Source: CAD feature listing. Evaluate the final solid. Frame: model axes, mm. Face numbers are marked on the shaded views. Coordinates: 2 decimals unless noted, no trailing zeros. Write each loop counter-clockwise with the first axis right and the second up, starting at its lowest first coordinate (ties: lowest second). Pieces come first, ordered by that corner, then holes. Notation, with made-up numbers: M 77,75.25 L 115,75.25 A26 cw 115,106.25 Z; hole C -4,-28 d7. An arc over 180 degrees is marked long. One line per item, written item: value. Start each with the question number.
Item 1: Cut plane B-B, the plane z = 1. Output: boundary loops of the cut face in (x, y), then the cut area to 3 significant figures.
Item 2: Cut plane A-A, the plane z = -19. Output: boundary loops of the cut face in (x, y).
Item 3: Pin query (flat end, axial travel): P1, Ø12, axis at x = -16, z = -2, coming from the -Y side; P2, Ø10, axis at y = -15, z = -2, coming from the -X side; P3, Ø5, axis at x = 0, y = 0, coming from the -Z side. Return the tip coordinate at first contact, or that it passes through.
Item 4: Ray query, L1, parallel to Y at x = 0, z = 22; L2, parallel to X at y = 0, z = 21.25; L3, parallel to X at y = 0, z = 18.25. Return the intervals inside material, ascending. Write a range as from..to.
Item 5: Mould query, pull axis X, two halves, no side actions, for the marked faces 1, 2, 3 and 4. Classes: released by +X, released by -X, zero draft, split by the parting line, or undercut.
Item 6: Cut plane C-C, the plane z = 10.5. Output: boundary loops of the cut face in (x, y), then the cut area to 3 significant figures.
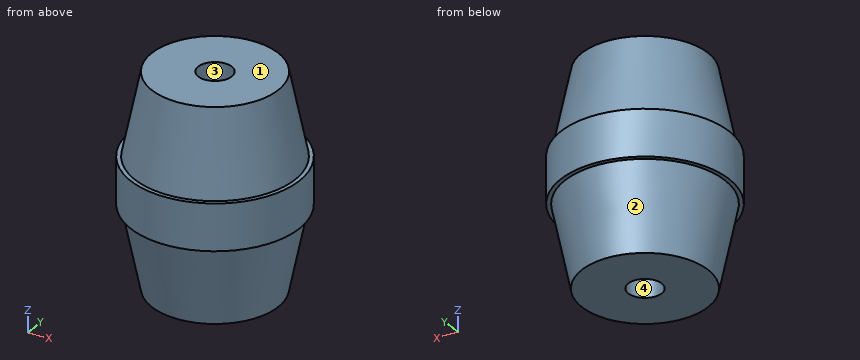
```python
from build123d import *

# Parameters (mm, degrees)
F4_D           = 8
F4_DEPTH       = 10
F4_TIP         = 2.4034424761
F4_ON_F2_D     = 8
F4_ON_F2_DEPTH = 10
F4_ON_F2_TIP   = 2.4034424761


with BuildPart() as f1:
    # F0 (on Front) → F1 (revolve)
    with BuildSketch(Plane.XZ):
        Polygon((0, -25), (0, 25), (-15, 25), (-19, 5.5), (-20, 5.5), (-20, 0), (-20, -5.5), (-20, -5.5145598017), (-19, -5.5145598017), (-15, -25), align=None)
    revolve(axis=Axis((0, 0, 0), (0, 0, -1)))

    # F4
    with Locations(Plane(origin=(0, 0, -25), x_dir=(1, 0, 0), z_dir=(0, 0, -1))):
        with Locations((0, 0)):
            Hole(F4_D / 2, depth=F4_DEPTH)
            with Locations((0, 0, -(F4_DEPTH + F4_TIP / 2))):  # 118° drill point
                Cone(0, F4_D / 2, F4_TIP, mode=Mode.SUBTRACT)

    # F4 on F2
    with Locations(Plane.XY.offset(25)):
        with Locations((0, 0)):
            Hole(F4_ON_F2_D / 2, depth=F4_ON_F2_DEPTH)
            with Locations((0, 0, -(F4_ON_F2_DEPTH + F4_ON_F2_TIP / 2))):  # 118° drill point
                Cone(0, F4_ON_F2_D / 2, F4_ON_F2_TIP, mode=Mode.SUBTRACT)


solid = f1.part
```
From the geometry:
1. outline: C 0,0 d40
1. area: 1,260 mm²
2. outline: C 0,0 d32.46; hole C 0,0 d8
3. P1: stops at y = -17.32
3. P2: stops at x = -17.32
3. P3: stops at z = -14.1
4. L1: y = -15.62..-4, 4..15.62
4. L2: x = -15.77..-4, 4..15.77
4. L3: x = -16.38..-4, 4..16.38
5. face 1: zero draft
5. face 2: split by the parting line
5. face 3: undercut
5. face 4: undercut
6. outline: C 0,0 d35.95
6. area: 1,010 mm²
